```python
from build123d import *

# Parameters (mm, degrees)
F0_W      = 76.2
F0_H      = 152.4
F1_DEPTH  = 50.8
F2_R      = 5.08
F3_W      = 66.04
F3_H      = 10.080694
F4_DEPTH  = 25.4
F5_W      = 66.04
F5_H      = 12.7
F6_DEPTH  = 12.7
F7_W      = 19.05
F7_H      = 6.35
F8_DEPTH  = 103.886
F9_R      = 16.51
F10_DEPTH = 38.1
F11_R     = 25.4
F11_R_2   = 16.51
F12_DEPTH = 4.318


with BuildPart() as f1:
    # F0 (on Front) → F1 (new body)
    with BuildSketch(Plane.XZ):
        with Locations((49.800091, 58.736403)):
            Rectangle(F0_W, F0_H)
    extrude(amount=F1_DEPTH)

    # F2
    f2_edges = [f1.edges().sort_by_distance(p)[0] for p in [
        (49.800091, -50.8, 134.936403),
        (11.700091, -50.8, 58.736403),
        (49.800091, -50.8, -17.463597),
        (87.900091, -50.8, 58.736403),
        (11.700091, -25.4, -17.463597),
        (87.900091, -25.4, -17.463597),
        (49.800091, 0, -17.463597),
        (49.800091, 0, 134.936403),
        (11.700091, 0, 58.736403),
        (87.900091, 0, 58.736403),
        (11.700091, -25.4, 134.936403),
        (87.900091, -25.4, 134.936403),
    ]]
    fillet(f2_edges, radius=F2_R)

    # F3 (on face) → F4 (join)
    with BuildSketch(Plane.XZ.offset(50.8)):
        with Locations((49.800091, -7.34325)):
            Rectangle(F3_W, F3_H)
    extrude(amount=F4_DEPTH)

    # F5 (on face) → F6 (join)
    with BuildSketch(Plane.XY.offset(-2.302903)):
        with Locations((49.800091, -69.85)):
            Rectangle(F5_W, F5_H)
    extrude(amount=F6_DEPTH)

    # F7 (on face) → F8 (cut)
    with BuildSketch(Plane(origin=(0, 0, -12.383597), x_dir=(1, 0, 0), z_dir=(0, 0, -1))):
        with Locations((49.800091, 57.138579)):
            Rectangle(F7_W, F7_H)
    extrude(amount=-F8_DEPTH, mode=Mode.SUBTRACT)

    # F9 (on face) → F10 (join)
    with BuildSketch(Plane(origin=(0, 0, 0), x_dir=(-1, 0, 0), z_dir=(0, 1, 0))):
        with Locations((-49.800091, 79.056403)):
            Circle(F9_R)
    extrude(amount=F10_DEPTH)

    # F11 (on face) → F12 (join)
    with BuildSketch(Plane(origin=(0, 38.1, 0), x_dir=(-1, 0, 0), z_dir=(0, 1, 0))):
        with Locations((-49.800091, 79.056403)):
            Circle(F11_R)
        with Locations((-49.800091, 79.056403)):
            Circle(F11_R_2, mode=Mode.SUBTRACT)
    extrude(amount=-F12_DEPTH)


solid = f1.part
```
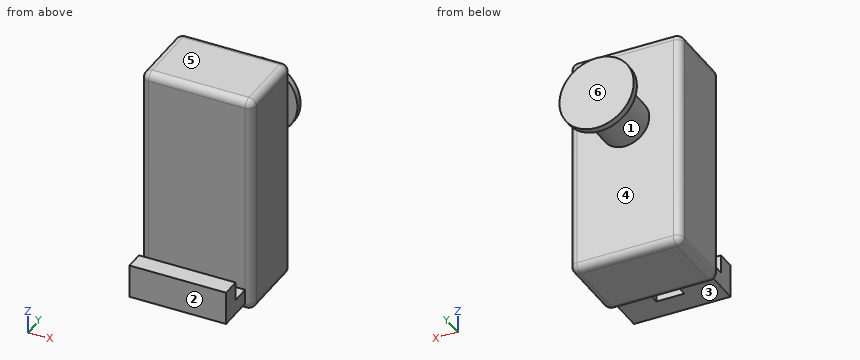
Geometry: final body of the model. Coordinates: model frame, mm. Face numbers are marked on the shaded views. A direction names the side the tool comes from. Give positions to 0.01 mm unless a question says otherwise; leave off trailing zeros. Write each loop counter-clockwise with the first axis right and the second up, starting at its lowest first coordinate (ties: lowest second). Pieces come first, ordered by that corner, then holes.
1. Draft query along Y for the marked faces 4, 5 and 6. Return one class per face: released by +Y, released by -Y, zero draft, split by the parting line, or undercut.
2. Line query: probe 1 along Z at (x, y) = (54, -51); probe 2 along Y at (x, z) = (19, 47.5); probe 3 along Y at (x, z) = (50, 73.5). Output: solid intervals per line, ascending.
3. Section query C-C, the plane x = 21. Return loops of the section in (y, z).
4. Section query D-D, the plane z = 98.5. Return loops of the section in (x, y).
5. Section query A-A, the plane x = 72.5. Return loops of the section in (y, z).
6. Pin query (flat end, axial travel): P1, Ø5, axis at x = 53, z = -9, coming from the +Y side; P2, Ø18, axis at y = -65, z = 0, coming from the +X side; P3, Ø14, axis at x = 62, y = -58, coming from the +Z side. Return the tip coordinate at first contact, or that it passes through.
7. Section query B-B, the plane z = 39. Return loops of the section in (x, y), then the cut area to 3 significant figures.
8. Reachability of the marked faces 1, 2 and 3 from +Z, -Z, +X, -X, +Y, -Y: full face, straight path, thin tool, end or side. Return the list, or none.
Computed:
1. face 4: undercut
1. face 5: zero draft
1. face 6: released by +Y
2. probe 1: z = -12.38 to -2.3
2. probe 2: y = -50.8 to 0
2. probe 3: y = -50.8 to 38.1
3. outline: (-76.2, -12.38) - (-50.8, -12.38) arc R5.08 ccw to (-45.72, -17.46) - (-5.08, -17.46) arc R5.08 ccw to (0, -12.38) - (0, 129.86) arc R5.08 ccw to (-5.08, 134.94) - (-45.72, 134.94) arc R5.08 ccw to (-50.8, 129.86) - (-50.8, -2.3) - (-63.5, -2.3) - (-63.5, 10.4) - (-76.2, 10.4) - close
4. outline: (11.7, -45.72) arc R5.08 ccw to (16.78, -50.8) - (82.82, -50.8) arc R5.08 ccw to (87.9, -45.72) - (87.9, -5.08) arc R5.08 ccw to (82.82, 0) - (16.78, 0) arc R5.08 ccw to (11.7, -5.08) - close; (33.46, 33.78) - (66.14, 33.78) - (66.14, 38.1) - (33.46, 38.1) - close
5. outline: (-76.2, -12.38) - (-50.8, -12.38) arc R5.08 ccw to (-45.72, -17.46) - (-5.08, -17.46) arc R5.08 ccw to (0, -12.38) - (0, 129.86) arc R5.08 ccw to (-5.08, 134.94) - (-45.72, 134.94) arc R5.08 ccw to (-50.8, 129.86) - (-50.8, -2.3) - (-63.5, -2.3) - (-63.5, 10.4) - (-76.2, 10.4) - close; (33.78, 67.66) - (38.1, 67.66) - (38.1, 90.45) - (33.78, 90.45) - close
6. P1: stops at y = 0
6. P2: stops at x = 82.82
6. P3: stops at z = 10.4
7. outline: (11.7, -45.72) arc R5.08 ccw to (16.78, -50.8) - (82.82, -50.8) arc R5.08 ccw to (87.9, -45.72) - (87.9, -5.08) arc R5.08 ccw to (82.82, 0) - (16.78, 0) arc R5.08 ccw to (11.7, -5.08) - close
7. area: 3,850 mm2
8. face 1: none
8. face 2: +Z, -Z, +X, -X, -Y
8. face 3: -Z, +X, -X, -Y
